Source: CAD feature listing. Evaluate the final solid. Frame: model axes, mm. A direction names the side the tool comes from. Give positions to 0.01 mm unless a question says otherwise; leave off trailing zeros. Order: outer loops, then holes, each group sorted by start corner. A loop starts at its lowest first (then second) coordinate and runs counter-clockwise, first axis right, second up. Notation, with made-up numbers: (-16, -2) -> (-12, -2) arc R19 cw to (-12, 16) -> close; hole circle Ø11 at (89, 32). An arc over 180 degrees is marked (long way). Use CSV: the item, a comma, the result in double quotes.
```python
from build123d import *

# Parameters (mm, degrees)
SKETCH1_R           = 17.5
SKETCH1_R_2         = 15.5
BOSS_EXTRUDE1_DEPTH = 240
SKETCH2_R           = 17.5
SKETCH2_R_2         = 16.65
BOSS_EXTRUDE2_DEPTH = 10
SKETCH3_R           = 17.5
SKETCH3_R_2         = 16.6
CUT_EXTRUDE1_DEPTH  = 10


with BuildPart() as part:
    # Sketch1 → Boss-Extrude1 (new body)
    with BuildSketch(Plane(origin=(0, 0, 0), x_dir=(1, 0, 0), z_dir=(0, 1, 0))):
        with Locations(Location((0, 0, 0), (0, 0, 270))):
            Circle(SKETCH1_R)
        with Locations(Location((0, 0, 0), (0, 0, 270))):
            Circle(SKETCH1_R_2, mode=Mode.SUBTRACT)
    extrude(amount=BOSS_EXTRUDE1_DEPTH)

    # Sketch2 → Boss-Extrude2 (add)
    with BuildSketch(Plane(origin=(0, 240, 0), x_dir=(1, 0, 0), z_dir=(0, 1, 0))):
        with Locations(Location((0, 0, 0), (0, 0, 270))):
            Circle(SKETCH2_R)
        with Locations(Location((0, 0, 0), (0, 0, 270))):
            Circle(SKETCH2_R_2, mode=Mode.SUBTRACT)
    extrude(amount=BOSS_EXTRUDE2_DEPTH)

    # Sketch3 → Cut-Extrude1 (cut)
    with BuildSketch(Plane.XZ):
        with Locations(Location((0, 0, 0), (0, 0, 270))):
            Circle(SKETCH3_R)
        with Locations(Location((0, 0, 0), (0, 0, 270))):
            Circle(SKETCH3_R_2, mode=Mode.SUBTRACT)
    extrude(amount=-CUT_EXTRUDE1_DEPTH, mode=Mode.SUBTRACT)


solid = part.part
```
1. Section query B-B on z = 8. Return loops of the section in (x, y).
Answer below:
outline,"(-15.56, 10) -> (-14.55, 10) -> (-14.55, 0) -> (-13.28, 0) -> (-13.28, 240) -> (-14.6, 240) -> (-14.6, 250) -> (-15.56, 250) -> close; (13.28, 0) -> (14.55, 0) -> (14.55, 10) -> (15.56, 10) -> (15.56, 250) -> (14.6, 250) -> (14.6, 240) -> (13.28, 240) -> close"
2. Pin query (flat end, axial travel): P1, Ø1.5, axis at y = 77.5, z = -12.5, coming from the -X side; P2, Ø18.5, axis at x = 0, z = 0, coming from the -Y side; P3, Ø1, axis at y = 122, z = 6, coming from the -X side; P4, Ø10, axis at y = 141.5, z = -5.5, coming from the +X side. Return the tip coordinate at first contact, or that it passes through.
Answer below:
P1,"stops at x = -12.97"
P2,"passes through"
P3,"stops at x = -16.61"
P4,"stops at x = 17.49"
3. Ray query, line 1 along X through (y, z) = (83, 0); line 2 along X through (y, z) = (245.25, 0); line 3 along Z through (x, y) = (-5, 183.5). Return the intervals inside material, ascending.
Answer below:
line 1,"x = -17.5 to -15.5, 15.5 to 17.5"
line 2,"x = -17.5 to -16.65, 16.65 to 17.5"
line 3,"z = -16.77 to -14.67, 14.67 to 16.77"
4. Mould query, pull axis X, two halves, no side actions, for faces 4 (the flat face through (7, 0, -14)), 5 (the cylindrical face through (-10.648, 128.32, -13.887)), 6 (the cylindrical face through (5, 244.93, 15.88)). Classes: released by +X, released by -X, zero draft, split by the parting line, or undercut.
Answer below:
face 4,"zero draft"
face 5,"split by the parting line"
face 6,"undercut"
5. Section query C-C on y = 32. Return loops of the section in (x, z).
Answer below:
outline,"circle Ø35 at (0, 0); hole circle Ø31 at (0, 0)"
6. Section query A-A on x = 0. Return loops of the section in (y, z), plus the area to 3 significant figures.
Answer below:
outline,"(0, -16.6) -> (10, -16.6) -> (10, -17.5) -> (250, -17.5) -> (250, -16.65) -> (240, -16.65) -> (240, -15.5) -> (0, -15.5) -> close; (0, 15.5) -> (240, 15.5) -> (240, 16.65) -> (250, 16.65) -> (250, 17.5) -> (10, 17.5) -> (10, 16.6) -> (0, 16.6) -> close"
area,"959 mm²"
7. Access query for faces 1 (the cylindrical face through (15.368, 118.32, -2.018)), 2 (the flat face through (-6.4, 10, -15.5)), 3 (the flat face through (-15, 240, 5)). Directions: +Z, -Z, +X, -X, +Y, -Y. A direction counts if a zero-diameter tool reaches every point of the face in a straight line with its end or side. Return the directions, or none.
Answer below:
face 1,"+Y, -Y"
face 2,"-Y"
face 3,"+Y"
